from build123d import *

# Parameters (mm, degrees)
BOSS_EXTRUDE1_DEPTH = 3.175
SKETCH2_R           = 3.3782
CUT_EXTRUDE1_DEPTH  = 70.922121857
SKETCH3_R           = 3.3782
CUT_EXTRUDE2_DEPTH  = 70.922121857
FILLET1_R           = 25.4
FILLET2_R           = 3.175


with BuildPart() as part:
    # Sketch1 → Boss-Extrude1 (new, symmetric)
    with BuildSketch(Plane.XY):
        Polygon((-28.575, -12.7), (28.575, -12.7), (28.575, 63.5), (3.175, 63.5), (3.175, 12.7), (-28.575, 12.7), align=None)
    extrude(amount=BOSS_EXTRUDE1_DEPTH, both=True)

    # Sketch2 → Cut-Extrude1 (cut, through all)
    with BuildSketch(Plane.XY.offset(3.175)):
        with Locations((15.875, 25.4)):
            Circle(SKETCH2_R)
        with Locations((15.875, 50.8)):
            Circle(SKETCH2_R)
    extrude(amount=-CUT_EXTRUDE1_DEPTH, mode=Mode.SUBTRACT)

    # Sketch3 → Cut-Extrude2 (cut, through all)
    with BuildSketch(Plane.XY.offset(3.175)):
        with Locations((-14.2875, 0)):
            Circle(SKETCH3_R)
        with Locations((14.2875, 0)):
            Circle(SKETCH3_R)
    extrude(amount=-CUT_EXTRUDE2_DEPTH, mode=Mode.SUBTRACT)

    # Fillet1
    fillet1_edges = [part.edges().sort_by_distance(p)[0] for p in [
        (3.175, 12.7, 0),
    ]]
    fillet(fillet1_edges, radius=FILLET1_R)

    # Fillet2
    fillet2_edges = [part.edges().sort_by_distance(p)[0] for p in [
        (-28.575, 12.7, 0),
        (3.175, 63.5, 0),
    ]]
    fillet(fillet2_edges, radius=FILLET2_R)


solid = part.part
Model file for the job. Use its own axes, mm. A direction names the side the tool comes from. Round coordinates to 2 decimals unless told otherwise and drop trailing zeros. Loops run counter-clockwise (first coordinate to the right, second up) from the corner with the lowest first, then second, coordinate; pieces in that order, holes last. Notation, with made-up numbers: (-29, 51.5) - (26, 51.5) arc R25 cw to (26, 76.5) - close; hole circle Ø1 at (-9.5, -2). An arc over 180 degrees is marked (long way). Write each question's results on one line, items separated by ' | '.
(1) Saw through at D-D, the plane x = -23.5. List the corners of the cut face in (y, z) (3 decimals).
Answer below:
outline: (-12.7, -3.175) - (12.7, -3.175) - (12.7, 3.175) - (-12.7, 3.175) - close
(2) Mould opens along X. For faces 1 (the cylindrical face through (17.51, 1.01, 0.04)), 2 (the flat face through (6, 17, -3.175)), 3 (the cylindrical face through (4.08, 62.545, 0.044)) say: released by +X, released by -X, zero draft, split by the parting line, or undercut.
Answer below:
face 1: undercut | face 2: zero draft | face 3: released by -X
(3) Pin check, flat tips, straight feed: pin 1 (6 mm diameter, centred on x = 15.875, y = 50.8, fed in from -Z); pin 2 (3.5 mm diameter, centred on x = -23, z = 0, fed in from +Y). Stop position of each tip, or through.
Answer below:
pin 1: passes through | pin 2: stops at y = 12.72
(4) Saw through at A-A, the plane y = 50.8. List the corners of the cut face in (x, z) (3 decimals).
Answer below:
outline: (3.175, -3.175) - (12.497, -3.175) - (12.497, 3.175) - (3.175, 3.175) - close; (19.253, -3.175) - (28.575, -3.175) - (28.575, 3.175) - (19.253, 3.175) - close
(5) 3-axis set-ups, long thin cutter, end or side, ignore diameter. For faces 4 (the cylindrical face through (17.43, 22.4, 0.04)), 5 (the flat face through (3.175, 49, 0)): which of +Z, -Z, +X, -X, +Y, -Y reach the whole face in a straight line?
Answer below:
face 4: +Z, -Z | face 5: +Z, -Z, -X, +Y
(6) Wall check: L1, parallel to Y at x = 13.5, z = -2.75; L2, parallel to Y at x = 6, z = -2.5; L3, parallel to Y at x = -24, z = 1.75. Give the ranges that are in metal, low to high.
Answer below:
L1: y = -12.7 to -3.29, 3.29 to 23, 27.8 to 48.4, 53.2 to 63.5 | L2: y = -12.7 to 63.48 | L3: y = -12.7 to 12.7
(7) Saw through at B-B, the plane z = -1.75. Count the separate pieces of the cut face and the enclosed holes in it, then the cut area to 3 significant figures.
Answer below:
separate pieces: 1 | enclosed holes: 4 | area: 2,730 mm^2
(8) Saw through at C-C, the plane y = 0. List the corners of the cut face in (x, z) (3 decimals).
Answer below:
outline: (-28.575, -3.175) - (-17.666, -3.175) - (-17.666, 3.175) - (-28.575, 3.175) - close; (-10.909, -3.175) - (10.909, -3.175) - (10.909, 3.175) - (-10.909, 3.175) - close; (17.666, -3.175) - (28.575, -3.175) - (28.575, 3.175) - (17.666, 3.175) - close
